Autodesk Fusion 360 part; units mm, degrees
sketch "Sketch1" plane through (0, 0, 0) normal (0, 0, 1) x (1, 0, 0)
  circle A0 centre (0, 0) radius 4
  circle A1 centre (0, 0) radius 6.6
  dimension "d1" = 8
  dimension "d2" = 13.2
extrude "Extrude1" add sketch "Sketch1" along normal blind 9
chamfer "Chamfer1" distance 0.2 angle 45 1 edges at (-6.1534, -2.3867, 9)
chamfer "Chamfer2" distance 0.2 angle 45 1 edges at (-6.1534, -2.3867, 0)
Geometry check sheet. Reference: the model listing, model coordinates, mm. Give positions to 0.01 mm unless a question says otherwise; leave off trailing zeros. Order: outer loops, then holes, each group sorted by start corner. A loop starts at its lowest first (then second) coordinate and runs counter-clockwise, first axis right, second up.
1. Section check C-C, the plane z = 1. Enter the section's corners in (x, y).
2. Section check A-A, the plane y = 0. Enter the section's corners in (x, z), and give its area (3 significant figures).
3. Release check for a two-part mould opening along Y. For faces 1 (the face through (-3, -3, 0)), 2 (the face through (-4.864, -4.461, 4.44)), 3 (the face through (-0.867, 3.905, 4.437)) record: pulls with the +Y half, pulls with the -Y half, needs draft (parallel to the pull), parting line crosses it, or undercut.
4. Gauge pin test, flat end, axial feed: pin 1 Ø5 at (x, z) = (3.5, 1) entering from -Y. Record the tip position at first contact, or that the pin passes through.
5. Thickness scan on L1, parallel to Y at x = 0, z = 3; L2, parallel to Y at x = -3.25, z = 6; L3, parallel to X at y = 0.25, z = 0.75. Record the ranges inside material, lowest first.
Values follow:
1. outline: circle Ø13.2 at (0, 0); hole circle Ø8 at (0, 0)
2. outline: (-6.6, 0.2) - (-6.4, 0) - (-4, 0) - (-4, 9) - (-6.4, 9) - (-6.6, 8.8) - close; (4, 0) - (6.4, 0) - (6.6, 0.2) - (6.6, 8.8) - (6.4, 9) - (4, 9) - close
2. area: 46.7 mm2
3. face 1: needs draft
3. face 2: parting line crosses it
3. face 3: undercut
4. pin 1: stops at y = -6.52
5. L1: y = -6.6 to -4, 4 to 6.6
5. L2: y = -5.74 to -2.33, 2.33 to 5.74
5. L3: x = -6.6 to -3.99, 3.99 to 6.6
